Check sheet for the drawn part. Datum: minimum x, y, z corner. Units: mm. A direction names the side the tool comes from. Coordinates: 2 decimals unless noted, no trailing zeros. Loops run counter-clockwise (first coordinate to the right, second up) from the corner with the lowest first, then second, coordinate; pieces in that order, holes last. Notation, with made-up numbers: (-17, 45.25) -> (-6, 45.25) arc R14 cw to (-6, 57.25) -> close; hole circle Ø2 at (-20.5, 26). An arc over 180 degrees is marked (long way). Use CSV: the item, a comma, the result in double quotes. Start each with the question number.
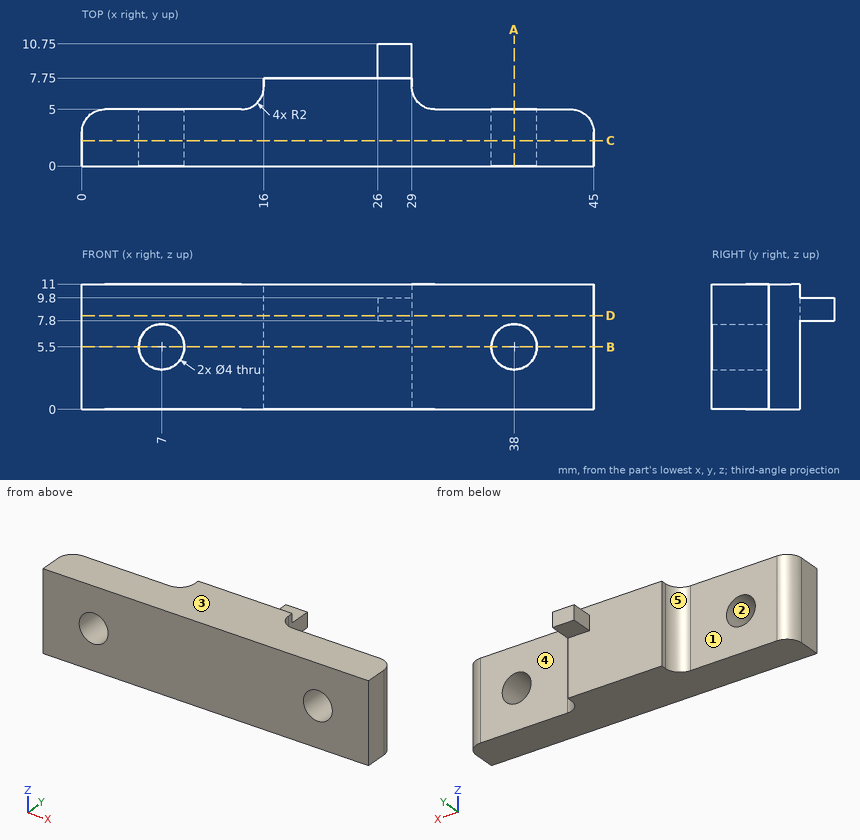
1. Cross-section at C-C, the plane y = 2.25. Record the boundary of the cut face in (x, z), plus the area to 3 significant figures.
2. Cross-section at A-A, the plane x = 38. Record the boundary of the cut face in (y, z).
3. Cross-section at D-D, the plane z = 8.25. Record the boundary of the cut face in (x, y), plus the area to 3 significant figures.
4. Scan lines: line 1 (X direction, y = 1.55, z = 5.5); line 2 (Z direction, x = 38, y = 3.3); line 3 (X direction, y = 0.75, z = 4.5). Record each from-to range of solid material in increasing order.
5. Depth check by flat-ended pin: pin 1 (0.9 mm diameter, centred on x = 27.5, y = 8.5, fed in from +Z); pin 2 (6 mm diameter, centred on y = 9, z = 5, fed in from +X); pin 3 (4.5 mm diameter, centred on x = 7, z = 5.5, fed in from +Y). Enter the tip coordinate at first touch or a pass-through.
6. Release check for a two-part mould opening along Z. For the marked faces 1, 2 and 3 record: released by +Z, released by -Z, zero draft, split by the parting line, or undercut.
7. Set-up check for the marked faces 4 and 5: record each of +Z, -Z, +X, -X, +Y, -Y from which the full face is reachable in a straight line by a thin tool's end or side.
8. Cross-section at B-B, the plane z = 5.5. Record the boundary of the cut face in (x, y).
Solution:
1,outline,"(0, 0) -> (45, 0) -> (45, 11) -> (0, 11) -> close; hole circle Ø4 at (7, 5.5); hole circle Ø4 at (38, 5.5)"
1,area,"470 mm2"
2,outline,"(0, 0) -> (5, 0) -> (5, 3.5) -> (0, 3.5) -> close; (0, 7.5) -> (5, 7.5) -> (5, 11) -> (0, 11) -> close"
3,outline,"(0, 0) -> (45, 0) -> (45, 3) arc R2 ccw to (43, 5) -> (31, 5) arc R2 cw to (29, 7) -> (29, 10.75) -> (26, 10.75) -> (26, 7.75) -> (16, 7.75) -> (16, 7) arc R2 cw to (14, 5) -> (2, 5) arc R2 ccw to (0, 3) -> close"
3,area,"270 mm2"
4,line 1,"x = 0 to 5, 9 to 36, 40 to 45"
4,line 2,"z = 0 to 3.5, 7.5 to 11"
4,line 3,"x = 0 to 5.27, 8.73 to 36.27, 39.73 to 45"
5,pin 1,"stops at z = 9.8"
5,pin 2,"stops at x = 29.27"
5,pin 3,"stops at y = 5"
6,face 1,"zero draft"
6,face 2,"undercut"
6,face 3,"released by +Z"
7,face 4,"+Z, -Z, +X, +Y"
7,face 5,"+Z, -Z, -X, +Y"
8,outline,"(0, 0) -> (5, 0) -> (5, 5) -> (2, 5) arc R2 ccw to (0, 3) -> close; (9, 0) -> (36, 0) -> (36, 5) -> (31, 5) arc R2 cw to (29, 7) -> (29, 7.75) -> (16, 7.75) -> (16, 7) arc R2 cw to (14, 5) -> (9, 5) -> close; (40, 0) -> (45, 0) -> (45, 3) arc R2 ccw to (43, 5) -> (40, 5) -> close"
